```python
from build123d import *

# Parameters (mm, degrees)
F1_R         = 7.5
F2_DEPTH     = 6
F3_R         = 1
F4_T         = -2.4
F7_DEPTH     = 4.6
F9_DEPTH     = 1.4
F10_SIZE     = 0.5
F11_T1_DEPTH = 4.5650872514
F11_T3_DEPTH = 6.9781403955
F11_T5_DEPTH = 6.9781403955


# Not quite as in the source:
# - a fillet or chamfer that OpenCascade refuses, or shapes differently, is made with other operations: its cross-section is extruded or revolved along the edge and cut away or added


with BuildPart() as f2:
    # F1 (on offset) → F2 (new body)
    with BuildSketch(Plane.XZ.offset(13)):
        with Locations((-13, 13)):
            Circle(F1_R)
    extrude(amount=-F2_DEPTH)

    # F3
    f3_edges = [f2.edges().sort_by_distance(p)[0] for p in [
        (-20.5, -13, 13),
    ]]
    fillet(f3_edges, radius=F3_R)

    # F4
    f4_openings = [f2.faces().sort_by_distance(p)[0] for p in [
        (-13, -7, 13),
    ]]
    offset(amount=F4_T, openings=f4_openings)

    # F6 (on offset) → F7 (join, through all)
    with BuildSketch(Plane.XZ.offset(2.4)):
        with BuildLine():
            Line((-10, 17.1243181255), (-10, 18.4258639865))
            ThreePointArc((-10, 18.4258639865), (-13, 19.2), (-16, 18.4258639865))
            Line((-16, 18.4258639865), (-16, 17.1243181255))
            ThreePointArc((-16, 17.1243181255), (-13, 18.1), (-10, 17.1243181255))
        make_face()
        with BuildLine():
            ThreePointArc((-10, 8.8756818745), (-13, 7.9), (-16, 8.8756818745))
            Line((-16, 8.8756818745), (-16, 7.5741360135))
            ThreePointArc((-16, 7.5741360135), (-13, 6.8), (-10, 7.5741360135))
            Line((-10, 7.5741360135), (-10, 8.8756818745))
        make_face()
    extrude(amount=F7_DEPTH)

    # F8 (on offset) → F9 (join)
    with BuildSketch(Plane.XZ.offset(2.4)):
        with BuildLine():
            Line((-16, 8.8756818745), (-16, 6.3449267472))
            ThreePointArc((-16, 6.3449267472), (-13, 5.7), (-10, 6.3449267472))
            Line((-10, 6.3449267472), (-10, 8.8756818745))
            ThreePointArc((-10, 8.8756818745), (-13, 7.9), (-16, 8.8756818745))
        make_face()
        with BuildLine():
            Line((-10, 17.1243181255), (-10, 19.6550732528))
            ThreePointArc((-10, 19.6550732528), (-13, 20.3), (-16, 19.6550732528))
            Line((-16, 19.6550732528), (-16, 17.1243181255))
            ThreePointArc((-16, 17.1243181255), (-13, 18.1), (-10, 17.1243181255))
        make_face()
    extrude(amount=-F9_DEPTH)

    # F10
    f10_edges = [f2.edges().sort_by_distance(p)[0] for p in [
        (-13, -1, 5.7),
        (-13, -1, 20.3),
    ]]
    chamfer(f10_edges, length=F10_SIZE)

    # F11: fillet of radius 1 on 8 edges, made by hand

    # F11_s2 → F11_t1 (cut)
    with BuildSketch(Plane.XZ.offset(-0.3325436257)):
        with BuildLine():
            ThreePointArc((-10, 18.9741108125), (-10.1883780691, 19.5582938671), (-10.6825396825, 19.92238237))
            ThreePointArc((-10.6825396825, 19.92238237), (-10.3379125488, 19.7973002289), (-10, 19.6550732528))
            Line((-10, 19.6550732528), (-10, 18.9741108125))
        make_face()
        with BuildLine():
            ThreePointArc((-15.3174603175, 19.92238237), (-15.8116219309, 19.5582938671), (-16, 18.9741108125))
            Line((-16, 18.9741108125), (-16, 19.6550732528))
            ThreePointArc((-16, 19.6550732528), (-15.6620874512, 19.7973002289), (-15.3174603175, 19.92238237))
        make_face()
        with BuildLine():
            ThreePointArc((-10, 7.0258891875), (-10.1883780691, 6.4417061329), (-10.6825396825, 6.07761763))
            ThreePointArc((-10.6825396825, 6.07761763), (-10.3379125488, 6.2026997711), (-10, 6.3449267472))
            Line((-10, 6.3449267472), (-10, 7.0258891875))
        make_face()
        with BuildLine():
            ThreePointArc((-16, 7.0258891875), (-15.8116219309, 6.4417061329), (-15.3174603175, 6.07761763))
            ThreePointArc((-15.3174603175, 6.07761763), (-15.6620874512, 6.2026997711), (-16, 6.3449267472))
            Line((-16, 6.3449267472), (-16, 7.0258891875))
        make_face()
    extrude(amount=F11_T1_DEPTH, mode=Mode.SUBTRACT)

    # F11_s4 → F11_t3 (cut)
    with BuildSketch(Plane.XY.offset(14.6243181255)):
        with BuildLine():
            ThreePointArc((-10, -2), (-10.2928932188, -1.2928932188), (-11, -1))
            Line((-11, -1), (-10, -1))
            Line((-10, -1), (-10, -2))
        make_face()
        with BuildLine():
            ThreePointArc((-15, -1), (-15.7071067812, -1.2928932188), (-16, -2))
            Line((-16, -2), (-16, -1))
            Line((-16, -1), (-15, -1))
        make_face()
    extrude(amount=F11_T3_DEPTH, mode=Mode.SUBTRACT)

    # F11_s6 → F11_t5 (cut)
    with BuildSketch(Plane.XY.offset(4.397541479)):
        with BuildLine():
            ThreePointArc((-16, -2), (-15.7071067812, -1.2928932188), (-15, -1))
            Line((-15, -1), (-16, -1))
            Line((-16, -1), (-16, -2))
        make_face()
        with BuildLine():
            ThreePointArc((-10, -2), (-10.2928932188, -1.2928932188), (-11, -1))
            Line((-11, -1), (-10, -1))
            Line((-10, -1), (-10, -2))
        make_face()
    extrude(amount=F11_T5_DEPTH, mode=Mode.SUBTRACT)


solid = f2.part
```
For this review, take the finished solid that the model builds, in its own axes (mm). A direction names the side the tool comes from. Coordinates: 2 decimals unless noted, no trailing zeros. Order: outer loops, then holes, each group sorted by start corner. A loop starts at its lowest first (then second) coordinate and runs counter-clockwise, first axis right, second up. Notation, with made-up numbers: (78.25, 22.25) - (108.25, 22.25) arc R29 ccw to (108.25, 53.25) - close; hole circle Ø3 at (-25, 76). An arc over 180 degrees is marked (long way). Answer as a JSON object with one key per item and string values. Group by question number.
1. The part is to be moulded in two halves that separate along Y. For faces 6 (the cylindrical face through (-15.699, -1.285, 18.349)), 7 (the flat face through (-10, -5, 8)), 8 (the flat face through (-13, -2.4, 20)), 9 (the flat face through (-13, -13, 13)), say which applies: pulls with the +Y half, pulls with the -Y half, needs draft (parallel to the pull), parting line crosses it, or undercut.
2. We need section C-C on x = -13. State the section outline as (y, z) points.
3. For probe 1 along Z at (x, y) = (-13, -7.85); probe 2 along Z at (x, y) = (-7.5, -8.75); probe 3 along Y at (x, z) = (-13.25, 18), list the stretches that pass through material, from the lowest coordinate up.
4. We need section D-D on y = -9.75. State the section outline as (x, z) points, then the cut area to 3 significant figures.
5. For faces 1 (the cylindrical face through (-15.806, -1.991, 19.565)), 2 (the cylindrical face through (-10.27, -1.99, 6.34)), 3 (the cylindrical face through (-10.27, -1.99, 19.66)), 4 (the cylindrical face through (-13, -4.7, 19.2)), 5 (the flat face through (-16, -5, 8)), list the 3-axis set-ups (+Z, -Z, +X, -X, +Y, -Y) from which the entire face can be reached by the end or side of a thin tool; tool diameter is ignored.
6. We need section B-B on z = 13. State the section outline as (x, y) points.
7. We need section A-A on y = -5. State the section outline as (x, z) points.
8. Clearance check with flat-ended pins moving along their axes: P1, Ø5, axis at y = -5, z = 12.5, coming from the -X side; P2, Ø2, axis at y = -4.5, z = 7.5, coming from the +X side; P3, Ø2, axis at y = -4, z = 8, coming from the -X side; P4, Ø0.9, axis at x = -11.5, z = 20, coming from the -Y side. State where each tip first meets the part, or that it passes through.
Final values:
{
 "1": {"face 6": "pulls with the +Y half", "face 7": "needs draft", "face 8": "undercut", "face 9": "pulls with the -Y half"},
 "2": {"outline": "(-13, 6.5) arc R1 ccw to (-12, 5.5) - (-7, 5.5) - (-7, 6.8) - (-2.4, 6.8) - (-2.4, 5.7) - (-1.5, 5.7) - (-1, 6.2) - (-1, 7.9) - (-10.6, 7.9) - (-10.6, 18.1) - (-1, 18.1) - (-1, 19.8) - (-1.5, 20.3) - (-2.4, 20.3) - (-2.4, 19.2) - (-7, 19.2) - (-7, 20.5) - (-12, 20.5) arc R1 ccw to (-13, 19.5) - close"},
 "3": {"probe 1": "5.5 to 7.9, 18.1 to 20.5", "probe 2": "7.9 to 18.1", "probe 3": "-13 to -10.6"},
 "4": {"outline": "circle Ø15 at (-13, 13); hole circle Ø10.2 at (-13, 13)", "area": "95.0 mm²"},
 "5": {"face 1": "+Z, -X, +Y", "face 2": "-Z, +X, +Y", "face 3": "+Z, +X, +Y", "face 4": "+Z", "face 5": "+Z, -Z, -X, +Y"},
 "6": {"outline": "(-20.5, -12) arc R1 ccw to (-19.5, -13) - (-6.5, -13) arc R1 ccw to (-5.5, -12) - (-5.5, -7) - (-7.9, -7) - (-7.9, -10.6) - (-18.1, -10.6) - (-18.1, -7) - (-20.5, -7) - close"},
 "7": {"outline": "(-16, 7.57) arc R6.2 ccw to (-10, 7.57) - (-10, 8.88) arc R5.1 cw to (-16, 8.88) - close; (-16, 17.12) arc R5.1 cw to (-10, 17.12) - (-10, 18.43) arc R6.2 ccw to (-16, 18.43) - close"},
 "8": {"P1": "x = -20.5", "P2": "x = -10", "P3": "x = -16", "P4": "y = -12.98"}
}
